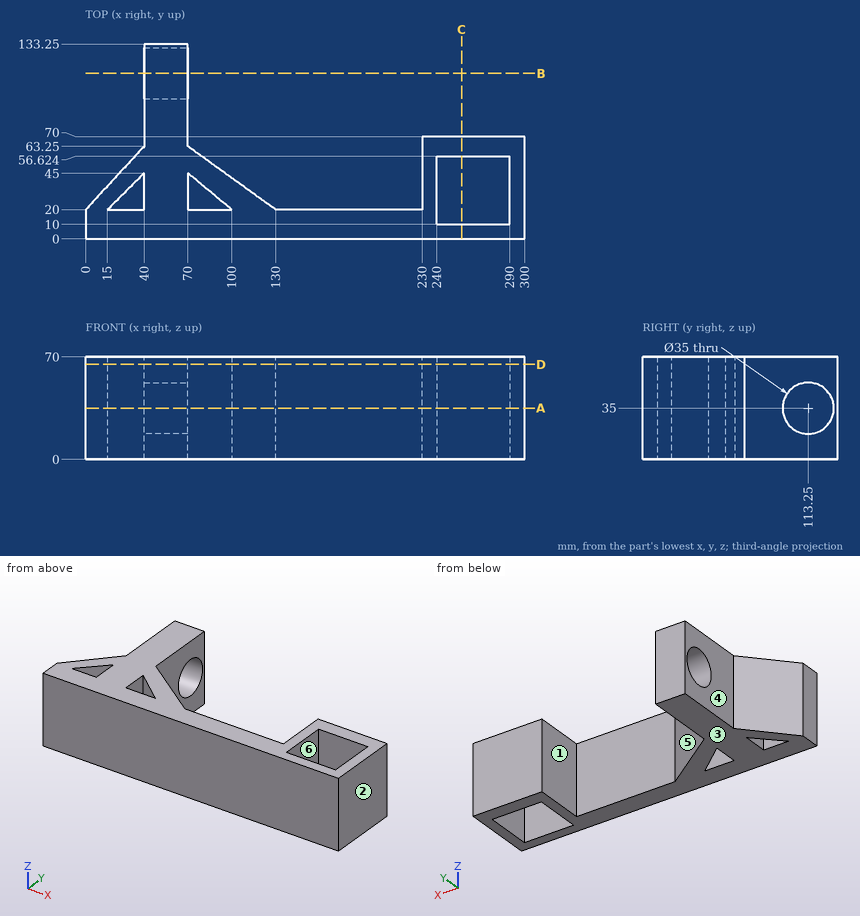
Geometry check sheet. Reference: drawing and pictorial views, mm from the part's lowest x, y, z. A direction names the side the tool comes from. Coordinates: 2 decimals unless noted, no trailing zeros. Write each loop counter-clockwise with the first axis right and the second up, starting at its lowest first coordinate (ties: lowest second). Pieces come first, ordered by that corner, then holes.
Item 1: Access from +Z, -Z, +X, -X, +Y, -Y to the whole of each face (thin tool, end or side, straight path). Record for the marked faces 4, 5 and 6.
Numbers:
face 4: +Z, -Z, -X, +Y
face 5: +Z, -Z, +Y
face 6: +Z, -Z
Item 2: Cross-section at B-B on y = 113.25. Record the boundary of the cut face in (x, z).
Numbers:
outline: (40, 0) - (70, 0) - (70, 17.5) - (40, 17.5) - close; (40, 52.5) - (70, 52.5) - (70, 70) - (40, 70) - close
Item 3: Scan lines: probe 1 along Y at (x, z) = (46.5, 35); probe 2 along Z at (x, y) = (46, 113); probe 3 along X at (y, z) = (66.5, 5). Record each from-to range of solid material in increasing order.
Numbers:
probe 1: y = 0 to 95.75, 130.75 to 133.25
probe 2: z = 0 to 17.5, 52.5 to 70
probe 3: x = 40 to 70, 230 to 300
Item 4: Cross-section at D-D on z = 65. Record the boundary of the cut face in (x, y), then the cut area to 3 significant figures.
Numbers:
outline: (0, 0) - (300, 0) - (300, 70) - (230, 70) - (230, 20) - (130, 20) - (70, 63.25) - (70, 133.25) - (40, 133.25) - (40, 63.25) - (0, 20) - close; hole (15, 20) - (40, 20) - (40, 45) - close; hole (70, 20) - (100, 20) - (70, 45) - close; hole (240, 10) - (290, 10) - (290, 56.62) - (240, 56.62) - close
area: 12,000 mm2
Item 5: Depth check by flat-ended pin: pin 1 Ø12 at (y, z) = (64.5, 9) entering from -X; pin 2 Ø8 at (y, z) = (118, 16) entering from +X; pin 3 Ø12.5 at (x, z) = (22.5, 31) entering from +Y. Enter the tip coordinate at first touch or a pass-through.
Numbers:
pin 1: stops at x = 35.61
pin 2: stops at x = 70
pin 3: stops at y = 51.09
Item 6: Mould release check, pull along X, two halves, no side actions. Record for the marked faces 1, 2 and 3: released by +X, released by -X, zero draft, split by the parting line, or undercut.
Numbers:
face 1: undercut
face 2: released by +X
face 3: zero draft
Item 7: Cross-section at A-A on z = 35. Record the boundary of the cut face in (x, y), then the cut area to 3 significant figures.
Numbers:
outline: (0, 0) - (300, 0) - (300, 70) - (230, 70) - (230, 20) - (130, 20) - (70, 63.25) - (70, 95.75) - (40, 95.75) - (40, 63.25) - (0, 20) - close; (40, 130.75) - (70, 130.75) - (70, 133.25) - (40, 133.25) - close; hole (15, 20) - (40, 20) - (40, 45) - close; hole (70, 20) - (100, 20) - (70, 45) - close; hole (240, 10) - (290, 10) - (290, 56.62) - (240, 56.62) - close
area: 11,000 mm2
Item 8: Cross-section at C-C on x = 257. Record the boundary of the cut face in (y, z).
Numbers:
outline: (0, 0) - (10, 0) - (10, 70) - (0, 70) - close; (56.62, 0) - (70, 0) - (70, 70) - (56.62, 70) - close
